Check sheet for the modelled part. Datum: model origin and axes. Units: mm. A direction names the side the tool comes from. Round coordinates to 2 decimals unless told otherwise and drop trailing zeros. Write each loop counter-clockwise with the first axis right and the second up, starting at its lowest first coordinate (ties: lowest second). Pieces come first, ordered by that corner, then holes.
Item 1: Material ranges on line 1 along Y through (x, z) = (0, 2.4); line 2 along Y through (x, z) = (2.75, 15); line 3 along Y through (x, z) = (-6.5, 19), recorded low to high.
Item 2: Release check for a two-part mould opening along X. For faces 1 (the cylindrical face through (0.358, -11.273, 2.465)), 2 (the flat face through (0, 40, 2)), 3 (the flat face through (-10, 10.4, 4.8)) record: pulls with the +X half, pulls with the -X half, needs draft (parallel to the pull), parting line crosses it, or undercut.
Item 3: Set-up check for faces 4 (the flat face through (0, 30, 5)), 5 (the cylindrical face through (0.358, 36.727, 2.465)), 6 (the flat face through (-6.807, 30.14, 17.325)), 7 (the flat face through (0, -10, 5)), 8 (the flat face through (-2, 0, 17)): record each of +Z, -Z, +X, -X, +Y, -Y from which the full face is reachable in a straight line by a thin tool's end or side.
Item 4: Section check A-A, the plane z = 27.5. Record the cut outline in (x, y), plus the area to 3 significant figures.
Item 5: Section check D-D, the plane z = 20. Record the cut outline in (x, y), plus the area to 3 significant figures.
Item 6: Section check C-C, the plane x = 0. Record the cut outline in (y, z).
Item 7: Depth check by flat-ended pin: pin 1 (1.5 mm diameter, centred on x = 3.5, z = 8.5, fed in from -Y); pin 2 (6 mm diameter, centred on x = 0.5, y = 8, fed in from +Z); pin 3 (6.5 mm diameter, centred on x = 0, z = 20, fed in from +Y). Enter the tip coordinate at first touch or a pass-through.
Item 8: Section check B-B, the plane y = -14. Record the cut outline in (x, z).
from build123d import *

# Parameters (mm, degrees)
F1_DEPTH  = 30
F2_W      = 20
F2_H      = 25
F3_DEPTH  = 25
F5_W      = 12
F5_H      = 25
F6_DEPTH  = 17
F7_D      = 5.5
F7_DEPTH  = 40.001
F9_D      = 5.5
F10_W     = 12
F10_H     = 25
F11_DEPTH = 17
F13_D     = 5.5


with BuildPart() as f1:
    # F0 (on Top) → F1 (new body)
    with BuildSketch(Plane.XY):
        Polygon((-10, 20), (-10, 0), (-10, -20), (10, -20), (10, 0), (10, 20), (10, 40), (-10, 40), align=None)
    extrude(amount=F1_DEPTH)

    # F2 (on face) → F3 (cut)
    with BuildSketch(Plane(origin=(-10, 0, 0), x_dir=(0, -1, 0), z_dir=(-1, 0, 0))):
        Polygon((-40, 5), (-20, 30), (-40, 30), align=None)
        with Locations((-10, 17.5)):
            Rectangle(F2_W, F2_H)
        Polygon((20, 30), (0, 30), (20, 5), align=None)
    extrude(amount=-F3_DEPTH, mode=Mode.SUBTRACT)

    # F5 (on face) → F6 (cut)
    with BuildSketch(Plane(origin=(0, 40, 0), x_dir=(-1, 0, 0), z_dir=(0, 1, 0))):
        with Locations((0, 17.5)):
            Rectangle(F5_W, F5_H)
    extrude(amount=-F6_DEPTH, mode=Mode.SUBTRACT)

    # F7 (through all, one way)
    with BuildSketch(Plane(origin=(0, 0, 0), x_dir=(-1, 0, 0), z_dir=(0, -1, 0))):
        with Locations((0, -20)):
            Circle(F7_D / 2)
    extrude(amount=-F7_DEPTH, mode=Mode.SUBTRACT)

    # F9 (through all)
    with Locations(Plane(origin=(0, 20, 0), x_dir=(1, 0, 0), z_dir=(0, 1, 0))):
        with Locations((0, -20)):
            Hole(F9_D / 2)

    # F10 (on face) → F11 (cut)
    with BuildSketch(Plane.XZ.offset(20)):
        with Locations((0, 17.5)):
            Rectangle(F10_W, F10_H)
    extrude(amount=-F11_DEPTH, mode=Mode.SUBTRACT)

    # F13 (through all)
    with Locations(Plane.XY.offset(5)):
        with Locations((0, 34), (0, -14)):
            Hole(F13_D / 2)


solid = f1.part
Values found:
1. line 1: y = -20 to -16.75, -11.25 to 31.25, 36.75 to 40
1. line 2: y = -3 to 0, 20 to 23
1. line 3: y = -8.8 to 0, 20 to 28.8
2. face 1: undercut
2. face 2: needs draft
2. face 3: pulls with the -X half
3. face 4: +Z, +Y
3. face 5: +Z, -Z
3. face 6: +Z, +X, -X, +Y
3. face 7: +Z, -Y
3. face 8: +Z, +X, -X
4. outline: (-10, -2) - (10, -2) - (10, 0) - (-10, 0) - close; (-10, 20) - (10, 20) - (10, 22) - (-10, 22) - close
4. area: 80.0 mm2
5. outline: (-10, -8) - (-6, -8) - (-6, -3) - (-2.75, -3) - (-2.75, 0) - (-10, 0) - close; (-10, 20) - (-2.75, 20) - (-2.75, 23) - (-6, 23) - (-6, 28) - (-10, 28) - close; (2.75, -3) - (6, -3) - (6, -8) - (10, -8) - (10, 0) - (2.75, 0) - close; (2.75, 20) - (10, 20) - (10, 28) - (6, 28) - (6, 23) - (2.75, 23) - close
5. area: 167 mm2
6. outline: (-20, 0) - (-16.75, 0) - (-16.75, 5) - (-20, 5) - close; (-11.25, 0) - (31.25, 0) - (31.25, 5) - (23, 5) - (23, 17.25) - (20, 17.25) - (20, 5) - (0, 5) - (0, 17.25) - (-3, 17.25) - (-3, 5) - (-11.25, 5) - close; (-3, 22.75) - (0, 22.75) - (0, 30) - (-3, 26.25) - close; (20, 22.75) - (23, 22.75) - (23, 26.25) - (20, 30) - close; (36.75, 0) - (40, 0) - (40, 5) - (36.75, 5) - close
7. pin 1: stops at y = -3
7. pin 2: stops at z = 5
7. pin 3: stops at y = 23
8. outline: (-10, 0) - (-2.75, 0) - (-2.75, 5) - (-6, 5) - (-6, 12.5) - (-10, 12.5) - close; (2.75, 0) - (10, 0) - (10, 12.5) - (6, 12.5) - (6, 5) - (2.75, 5) - close
